For this review, take the finished solid that the model builds, in its own axes (mm). A direction names the side the tool comes from. Round coordinates to 2 decimals unless told otherwise and drop trailing zeros. Loops run counter-clockwise (first coordinate to the right, second up) from the corner with the lowest first, then second, coordinate; pieces in that order, holes last.
1) Take a section at B-B (z = 65). State the section outline as (x, y) points, then the cut area to 3 significant figures.
2) Tool access review of faces 4 (the flat face through (0, 15, 39)), 5 (the cylindrical face through (6.3, 12.5, 65.1)): name each direction out of +Z, -Z, +X, -X, +Y, -Y from which nothing blocks a thin tool from reaching the whole face with its end or side.
3) Wall thickness on L1, parallel to Z at x = 8.25, y = 15; L2, parallel to Y at x = 8.25, z = 65; L3, parallel to Y at x = -8, z = 49: over which ranges is each line inside the solid? List them lowest first.
4) Take a section at C-C (z = 37.5). State the section outline as (x, y) points.
5) Insertion check: pin 1 (5 mm diameter, centred on y = 18, z = 51.5, fed in from -X); pin 2 (1.5 mm diameter, centred on x = -8, z = 65, fed in from +Y); pin 3 (6 mm diameter, centred on y = 15, z = 15.02, fed in from -X). Each pin has a flat end and moves straight along its axis. Give the tip position at first contact, or say it passes through.
6) Take a section at A-A (y = 15). State the section outline as (x, z) points, then the cut area to 4 significant figures.
7) Take a section at D-D (x = -7). State the section outline as (y, z) points.
8) Mouldability with a two-part tool opening along Z and no side actions: class faces 1 (the flat face through (2, 12, 0)), 2 (the conical face through (2.38, 17.5, 15.81)), 3 (the flat face through (-5, 0, 39)) as pulls with the +Z half, pulls with the -Z half, needs draft (parallel to the pull), parting line crosses it, or undercut.
```python
from build123d import *

# Parameters (mm, degrees)
F1_DEPTH       = 80
F3_D           = 5
F3_CSINK_D     = 10
F3_CSINK_ANGLE = 90


with BuildPart() as f1:
    # F0 (on Top) → F1 (new body)
    with BuildSketch(Plane.XY):
        with BuildLine():
            Line((10, 0), (10, 30))
            Line((10, 30), (5, 30))
            ThreePointArc((5, 30), (1.464466, 28.535534), (0, 25))
            Line((0, 25), (0, 5))
            Line((0, 5), (0, 0))
            Line((0, 0), (10, 0))
        make_face()
        with BuildLine():
            Line((-19.651743, 0), (0, 0))
            Line((0, 0), (0, 5))
            Line((0, 5), (-14.651743, 5))
            ThreePointArc((-14.651743, 5), (-18.187277, 3.535534), (-19.651743, 0))
        make_face()
    extrude(amount=F1_DEPTH)

    # F3 (through all)
    with Locations(Plane(origin=(0, 0, 0), x_dir=(0, -1, 0), z_dir=(-1, 0, 0))):
        with Locations((-15, 15.017683), (-15, 65)):
            CounterSinkHole(F3_D / 2, F3_CSINK_D / 2, counter_sink_angle=F3_CSINK_ANGLE)


solid = f1.part
```
Response:
1. outline: (-19.65, 0) - (10, 0) - (10, 12.5) - (2.5, 12.5) - (0, 10) - (0, 5) - (-14.65, 5) arc R5 ccw to start; (0, 20) - (2.5, 17.5) - (10, 17.5) - (10, 30) - (5, 30) arc R5 ccw to (0, 25) - close
1. area: 331 mm2
2. face 4: +Z, -Z, -X, +Y
2. face 5: +X, -X
3. L1: z = 0 to 12.52, 17.52 to 62.5, 67.5 to 80
3. L2: y = 0 to 12.5, 17.5 to 30
3. L3: y = 0 to 5
4. outline: (-19.65, 0) - (10, 0) - (10, 30) - (5, 30) arc R5 ccw to (0, 25) - (0, 5) - (-14.65, 5) arc R5 ccw to start
5. pin 1: stops at x = 0
5. pin 2: stops at y = 5
5. pin 3: stops at x = 2
6. outline: (0, 0) - (10, 0) - (10, 12.52) - (2.5, 12.52) - (0, 10.02) - close; (0, 20.02) - (2.5, 17.52) - (10, 17.52) - (10, 62.5) - (2.5, 62.5) - (0, 60) - close; (0, 70) - (2.5, 67.5) - (10, 67.5) - (10, 80) - (0, 80) - close
6. area: 687.5 mm2
7. outline: (0, 0) - (5, 0) - (5, 80) - (0, 80) - close
8. face 1: pulls with the -Z half
8. face 2: undercut
8. face 3: needs draft
